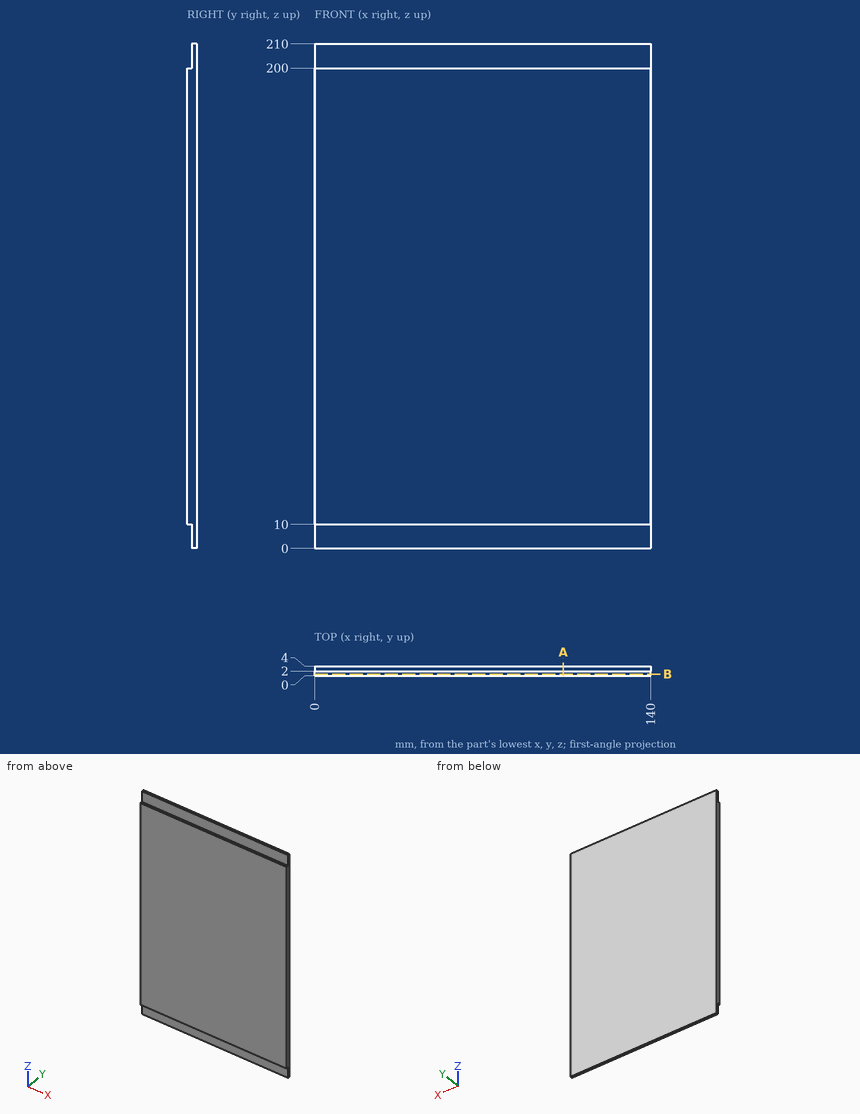
Geometry: see drawing. Coordinates: mm, zero at the bounding-box minimum. Give positions to 0.01 mm unless a question says otherwise; leave off trailing zeros. Write each loop counter-clockwise with the first axis right and the second up, starting at its lowest first coordinate (ties: lowest second). Pieces come first, ordered by that corner, then holes. Notation, with made-up numbers: (36, 89.25) - (56, 89.25) arc R23 ccw to (56, 116.25) - close; hole circle Ø5 at (-26.75, 26). An arc over 180 degrees is marked (long way). Return JSON: item names as keys, results as strings. Group by question number.
1) Line query: line 1 (Z direction, x = 59.5, y = 1.9); line 2 (Y direction, x = 40, z = 201). Output: solid intervals per line, ascending.
2) First-contact query: P1, Ø1, axis at x = 57.5, y = 1, coming from the -Z side; P2, Ø11, axis at x = 98, z = 207, coming from the -Y side; P3, Ø0.6, axis at x = 78, y = 1.5, coming from the +Z side. Flat tips, straight axial feed; report the tip coordinate or a pass-through.
3) Section B-B on y = 0.8. Return the cut outline in (x, z), plus the area to 3 significant figures.
4) Section A-A on x = 103.5. Return the cut outline in (y, z), plus the area to 3 significant figures.
Filled in:
{
 "1": {"line 1": "z = 10 to 200", "line 2": "y = 2 to 4"},
 "2": {"P1": "stops at z = 10", "P2": "stops at y = 2", "P3": "stops at z = 200"},
 "3": {"outline": "(0, 10) - (140, 10) - (140, 200) - (0, 200) - close", "area": "26,600 mm^2"},
 "4": {"outline": "(0, 10) - (2, 10) - (2, 0) - (4, 0) - (4, 210) - (2, 210) - (2, 200) - (0, 200) - close", "area": "800 mm^2"}
}
